Autodesk Inventor part; units mm, degrees
ref_plane "YZ Plane" through (0, 0, 0) normal (1, 0, 0) x (0, 1, 0)
ref_plane "XZ Plane" through (0, 0, 0) normal (0, 1, 0) x (-1, 0, 0)
ref_plane "XY Plane" through (0, 0, 0) normal (0, 0, 1) x (1, 0, 0)
sketch "草图1" plane through (0, 0, 0) normal (0, 0, 1) x (1, 0, 0)
  circle A0 centre (-65, 0.3085) radius 15
  circle A1 centre (65, 0.3085) radius 15
  arc A2 (-44.698, 14.8971) -> (-45.3152, -15.1029) centre (-65, 0.3085) ccw
  arc A3 (45.3152, -15.1029) -> (44.698, 14.8971) centre (65, 0.3085) ccw
  line L0 (0, 0) -> (0, 60.3628)
  line L1 (0, 0) -> (-51.6716, 0)
  line L2 (-44.698, 14.8971) -> (44.698, 14.8971)
  line L3 (45.3152, -15.1029) -> (-45.3152, -15.1029)
  line L4 (-44.698, 14.8971) -> (45.3152, -15.1029) construction
  line L5 (44.698, 14.8971) -> (-45.3152, -15.1029) construction
  dimension "d0" = 30
  dimension "d1" = 30
  dimension "d2" = 50
  dimension "d3" = 50
  dimension "d4" = 65
  dimension "d6" = 65
  dimension "d9" = 30
extrude "拉伸1" add sketch "草图1" along normal blind 10
properties part number "ConnectBar" material "钢，高强度，低合金"
Input: part model. Units: mm. Frame: model coordinates. A direction names the side the tool comes from. Round coordinates to 2 decimals unless told otherwise and drop trailing zeros. Loops run counter-clockwise (first coordinate to the right, second up) from the corner with the lowest first, then second, coordinate; pieces in that order, holes last. Notation, with made-up numbers: M 60.5,41 L 102.5,41 A15 ccw 102.5,45 Z; hole C 81.5,54.25 d1. An arc over 180 degrees is marked long. Answer in a Markdown table with one row per item. Add a question column.
1. Ray query, probe 1 along X at (y, z) = (0, 1); probe 2 along Y at (x, z) = (-65, 7); probe 3 along X at (y, z) = (7.5, 1.5). Return the intervals inside material, ascending.
2. Section C-C (z = 5.25). Output: boundary loops of the cut face in (x, y).
3. Set-up query: faces 3 (the face through (-1, 14.897, 5)), 4 (the face through (-79.985, -0.351, 4.93)), 5 (the face through (1, -15.103, 5)). Return all of +Z, -Z, +X, -X, +Y, -Y with unobstructed straight access to the full face (end or side cutting, diameter ignored); none if empty.
4. Contact query for flat-ended pins moving along their axis: pin 1 (5 mm diameter, centred on x = 7, z = 4, fed in from +Y); pin 2 (1.5 mm diameter, centred on y = -1.5, z = 6, fed in from +X); pin 3 (2 mm diameter, centred on y = -16.5, z = 9, fed in from -X). Output: stop coordinate, or through.
5. Section A-A (x = 65). Output: boundary loops of the cut face in (y, z), and give its area (3 significant figures).
6. Section B-B (y = -19.5). Output: boundary loops of the cut face in (x, z), and give its area (3 significant figures).
7. Mould query, pull axis X, two halves, no side actions, for faces 1 (the face through (-1, 1, 10)), 2 (the face through (50.015, -0.351, 4.93)). Classes: released by +X, released by -X, zero draft, split by the parting line, or undercut.
8. Section D-D (y = 11). Output: boundary loops of the cut face in (x, z).
Values follow:
| question | item | result |
|---|---|---|
| 1 | probe 1 | -90 to -80, -50 to 50, 80 to 90 |
| 1 | probe 2 | -24.69 to -14.69, 15.31 to 25.31 |
| 1 | probe 3 | -88.94 to -78.16, -51.84 to 51.84, 78.16 to 88.94 |
| 2 | outline | M -45.32,-15.1 L 45.32,-15.1 A25 ccw long 44.7,14.9 L -44.7,14.9 A25 ccw long Z; hole C -65,0.31 d30; hole C 65,0.31 d30 |
| 3 | face 3 | +Z, -Z, +Y |
| 3 | face 4 | +Z, -Z |
| 3 | face 5 | +Z, -Z, -Y |
| 4 | pin 1 | y = 14.9 |
| 4 | pin 2 | x = 89.98 |
| 4 | pin 3 | x = -84.37 |
| 5 | outline | M -24.69,0 L -14.69,0 L -14.69,10 L -24.69,10 Z; M 15.31,0 L 25.31,0 L 25.31,10 L 15.31,10 Z |
| 5 | area | 200 mm^2 |
| 6 | outline | M -80.25,0 L -49.75,0 L -49.75,10 L -80.25,10 Z; M 49.75,0 L 80.25,0 L 80.25,10 L 49.75,10 Z |
| 6 | area | 610 mm^2 |
| 7 | face 1 | zero draft |
| 7 | face 2 | undercut |
| 8 | outline | M -87.6,0 L -75.52,0 L -75.52,10 L -87.6,10 Z; M -54.48,0 L 54.48,0 L 54.48,10 L -54.48,10 Z; M 75.52,0 L 87.6,0 L 87.6,10 L 75.52,10 Z |
